CAD build for the part. Positions are in the model's coordinates, mm. Coordinates: 2 decimals unless noted, no trailing zeros. Write each loop counter-clockwise with the first axis right and the second up, starting at its lowest first coordinate (ties: lowest second). Pieces come first, ordered by that corner, then holes. Notation, with made-up numbers: M 21,26.5 L 80,26.5 A15 cw 80,45.5 Z; hole C -8,6 d4. An arc over 180 degrees is marked long. Answer as CSV lines item,"result". Start each with the question number.
```python
from build123d import *

# Parameters (mm, degrees)
F0_R     = 36.957
F1_DEPTH = 172.4406
F4_R     = 5.08


with BuildPart() as f1:
    # F0 (on Top) → F1 (new body)
    with BuildSketch(Plane.XY):
        Circle(F0_R)
    extrude(amount=F1_DEPTH)

    # F2 (on Front) → F3 (revolve)
    with BuildSketch(Plane.XZ):
        with BuildLine():
            Line((0, 172.4406), (36.957, 172.4406))
            ThreePointArc((36.957, 172.4406), (36.417433, 174.497665), (34.937665, 176.02506))
            ThreePointArc((34.937665, 176.02506), (33.979759, 176.943029), (33.5026, 178.181))
            Line((33.5026, 178.181), (34.937665, 180.924344))
            ThreePointArc((34.937665, 180.924344), (35.249759, 182.194272), (34.937665, 183.4642))
            Line((34.937665, 183.4642), (0, 183.4642))
            Line((0, 183.4642), (0, 172.4406))
        make_face()
    revolve(axis=Axis((0, 0, 177.9524), (0, 0, -1)))

    # F4
    f4_edges = [f1.edges().sort_by_distance(p)[0] for p in [
        (-36.957, 0, 0),
    ]]
    fillet(f4_edges, radius=F4_R)


solid = f1.part
```
1) Two-plate mould, pull along Z, no slides. Class faces 1 (the cylindrical face through (-4.811, 36.643, 87.589)), 2 (the flat face through (0, 0, 183.464)), 3 (the conical face through (15.5, 29.8, 178.35)): pulls with the +Z half, pulls with the -Z half, needs draft (parallel to the pull), parting line crosses it, or undercut.
2) Pin check, flat tips, straight feed: P1, Ø4, axis at y = 8, z = 69, coming from the -X side; P2, Ø5, axis at x = -13.5, z = 25, coming from the +Y side; P3, Ø2, axis at y = 8.5, z = 103.5, coming from the +X side. Stop position of each tip, or through.
3) Band-saw the part on A-A, the plane z = 164. List the corners of the cut face in (x, y).
4) Probe L1, parallel to X at y = 12, z = 28.5; L2, parallel to Z at x = -19, y = -28; L3, parallel to Z at x = 23, y = 24. List the from-to ranges inside material, lowest first. Write a range as [from, to].
Result sheet:
1,face 1,"needs draft"
1,face 2,"pulls with the +Z half"
1,face 3,"undercut"
2,P1,"stops at x = -36.47"
2,P2,"stops at y = 35.28"
2,P3,"stops at x = 36.19"
3,outline,"C 0,0 d73.91"
4,L1,"x = [-34.95, 34.95]"
4,L2,"z = [0.39, 177.18], [178.82, 183.46]"
4,L3,"z = [0.19, 183.46]"
